Input: dimensioned drawing with shaded views. Units: mm. Origin: part minimum x, y, z. Round coordinates to 2 decimals unless told otherwise and drop trailing zeros. Order: outer loops, then holes, each group sorted by start corner. A loop starts at its lowest first (then second) coordinate and runs counter-clockwise, first axis right, second up. Notation, with made-up numbers: (43.5, -9) - (94.5, -9) arc R22 ccw to (94.5, 29) - close; hole circle Ø11 at (65, 17). An arc over 180 degrees is marked (long way). Put each result on its own line as item: value. Start each with the question number.
(1) Pull-direction query (Z, two-part tool) for the marked faces 1 and 2; classes: released by +Z, released by -Z, zero draft, split by the parting line, or undercut.
(2) Material intervals for L1, parallel to Z at x = 85, y = 3.65; L2, parallel to X at y = 3.1, z = 8.5; L3, parallel to X at y = 1.85, z = 16, sorted ascending. Write a range as [from, to].
(3) Pin query (flat end, axial travel): P1, Ø2.5, axis at x = 5, z = 15, coming from the +Y side. Return the tip coordinate at first contact, or that it passes through.
(4) Section B-B (x = 85). Output: boundary loops of the cut face in (y, z), and give its area (3 significant figures).
(5) Section A-A (x = 15). Output: boundary loops of the cut face in (y, z), and give its area (3 significant figures).
(6) Section D-D (z = 10). Output: boundary loops of the cut face in (x, y), and give its area (3 significant figures).
(7) Section C-C (y = 3.45). Count the separate pieces of the cut face and the enclosed holes in it, and give its area (3 significant figures).
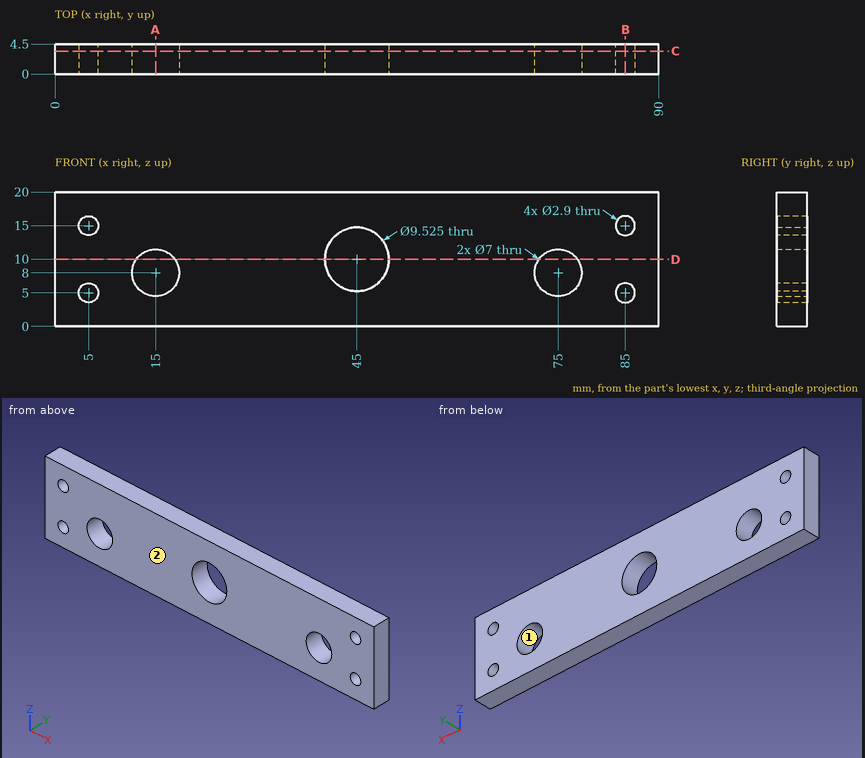
Checks:
1. face 1: undercut
1. face 2: zero draft
2. L1: z = [0, 3.55], [6.45, 13.55], [16.45, 20]
2. L2: x = [0, 11.54], [18.46, 40.48], [49.52, 71.54], [78.46, 90]
2. L3: x = [0, 3.95], [6.05, 83.95], [86.05, 90]
3. P1: passes through
4. outline: (0, 0) - (4.5, 0) - (4.5, 3.55) - (0, 3.55) - close; (0, 6.45) - (4.5, 6.45) - (4.5, 13.55) - (0, 13.55) - close; (0, 16.45) - (4.5, 16.45) - (4.5, 20) - (0, 20) - close
4. area: 63.9 mm²
5. outline: (0, 0) - (4.5, 0) - (4.5, 4.5) - (0, 4.5) - close; (0, 11.5) - (4.5, 11.5) - (4.5, 20) - (0, 20) - close
5. area: 58.5 mm²
6. outline: (0, 0) - (12.13, 0) - (12.13, 4.5) - (0, 4.5) - close; (17.87, 0) - (40.24, 0) - (40.24, 4.5) - (17.87, 4.5) - close; (49.76, 0) - (72.13, 0) - (72.13, 4.5) - (49.76, 4.5) - close; (77.87, 0) - (90, 0) - (90, 4.5) - (77.87, 4.5) - close
6. area: 310 mm²
7. separate pieces: 1
7. enclosed holes: 7
7. area: 1,630 mm²
